from build123d import *

# Parameters (mm, degrees)
F2_W     = 4.7625
F2_H     = 25.4
F3_DEPTH = 42.8635


with BuildPart() as f1:
    # F0 (on Front) → F1 (revolve)
    with BuildSketch(Plane.XZ):
        Polygon((-39.6875, 0), (-38.1, 0), (-38.1, 25.4), (0, 25.4), (0, 28.575), (-42.8625, 28.575), (-42.8625, 25.4), (-39.6875, 25.4), align=None)
    revolve(axis=Axis((0, 0, 14.2875), (0, 0, 1)))

    # F2 (on Front) → F3 (cut, through all)
    with BuildSketch(Plane.XZ):
        with Locations((0, 12.7)):
            Rectangle(F2_W, F2_H)
    extrude(amount=F3_DEPTH, mode=Mode.SUBTRACT)


solid = f1.part
Read the model definition and answer for the solid it produces. Units are mm, in the model's axes. Round coordinates to 2 decimals unless told otherwise and drop trailing zeros. Write each loop counter-clockwise with the first axis right and the second up, starting at its lowest first coordinate (ties: lowest second). Pieces come first, ordered by that corner, then holes. Notation, with made-up numbers: (-22, 68.5) - (22, 68.5) arc R14 ccw to (22, 93.5) - close; hole circle Ø1 at (17, 28.5). An arc over 180 degrees is marked (long way). One line per question, with ' | ' between items. Start each with the question number.
1. Section A-A (x = 0) is taken. Determine the outline of the cut face in (y, z) (1 decimal).
2. Find the intervals of material crossed by probe 1 along X at (y, z) = (0, 6.75); probe 2 along Z at (x, y) = (27.5, 17.5) (3 decimals); probe 3 along Y at (x, z) = (0, 18.25), in increasing order. Write a range as [from, to].
3. Section C-C (z = 4.75) is taken. Determine the outline of the cut face in (x, y) (1 decimal), and give its area (3 significant figures).
4. Section D-D (x = 29) is taken. Determine the outline of the cut face in (y, z) (3 decimals).
5. Section B-B (y = 24.5) is taken. Determine the outline of the cut face in (x, z) (3 decimals).
6. For a pull along Y with two mould halves and no side action, classify faces 1 (the face through (1, -1, 25.4)), 2 (the face through (-23.043, -36.142, 26.965)), 3 (the face through (-1, -1, 28.575)) as +Y half, -Y half, draft (parallel to the pull), parting line (faces both ways), or undercut.
7. Each of these flat-tipped pins is pushed along its axis until it touches: pin 1 (5 mm diameter, centred on x = 6, z = 4.5, fed in from +Y); pin 2 (10 mm diameter, centred on y = -4, z = 21, fed in from -X); pin 3 (6 mm diameter, centred on x = -29.5, z = 19.5, fed in from -Y); pin 4 (3 mm diameter, centred on x = 30, y = 33.5, fed in from -Z). Where does it stop, or does it pass through?
Filled in:
1) outline: (-42.9, 25.4) - (38.1, 25.4) - (38.1, 0) - (39.7, 0) - (39.7, 25.4) - (42.9, 25.4) - (42.9, 28.6) - (-42.9, 28.6) - close
2) probe 1: [-39.69, -38.1], [38.1, 39.69] | probe 2: [25.4, 28.575] | probe 3: [38.1, 39.69]
3) outline: (-2.4, -39.6) - (-2.4, -38) arc R38.1 cw (long way) to (2.4, -38) - (2.4, -39.6) arc R39.7 ccw (long way) to start | area: 380 mm²
4) outline: (-31.563, 25.4) - (-27.094, 25.4) - (-27.094, 0) - (-24.711, 0) - (-24.711, 25.4) - (24.711, 25.4) - (24.711, 0) - (27.094, 0) - (27.094, 25.4) - (31.563, 25.4) - (31.563, 28.575) - (-31.563, 28.575) - close
5) outline: (-35.17, 25.4) - (-31.223, 25.4) - (-31.223, 0) - (-29.178, 0) - (-29.178, 25.4) - (29.178, 25.4) - (29.178, 0) - (31.223, 0) - (31.223, 25.4) - (35.17, 25.4) - (35.17, 28.575) - (-35.17, 28.575) - close
6) face 1: undercut | face 2: parting line | face 3: draft
7) pin 1: y = 39.53 | pin 2: x = -42.83 | pin 3: y = -29.54 | pin 4: through
